Autodesk Inventor part; units mm, degrees
ref_plane "YZ Plane" through (0, 0, 0) normal (1, 0, 0) x (0, 1, 0)
ref_plane "XZ Plane" through (0, 0, 0) normal (0, 1, 0) x (-1, 0, 0)
ref_plane "XY Plane" through (0, 0, 0) normal (0, 0, 1) x (1, 0, 0)
sketch "Náčrt2" plane through (0, 0, 0) normal (0, 0, 1) x (1, 0, 0)
  line L0 (-2.8, -6) -> (2.8, -6)
  line L1 (2.8, -6) -> (2.8, 6)
  line L2 (2.8, 6) -> (-2.8, 6)
  line L3 (-2.8, 6) -> (-2.8, -6)
  line L4 (-2.8, -6) -> (2.8, 6) construction
  line L5 (2.8, -6) -> (-2.8, 6) construction
  circle A0 centre (0, 0) radius 1.5
  dimension "d0" = 5.6
  dimension "d1" = 12
  dimension "d2" = 3
extrude "Vysunutí1" add sketch "Náčrt2" along normal blind 2.75
fillet "Zaoblení1" radius 1.2 4 edges at (-2.8, 6, 1.375) (2.8, 6, 1.375) (2.8, -6, 1.375) (-2.8, -6, 1.375)
chamfer "Zkosení1" distance 0.2 angle 45 2 edges at (-1.5, 0, 2.75) (-1.5, 0, 0)
properties part number "rapoukServoWasherv0_3D tisk"
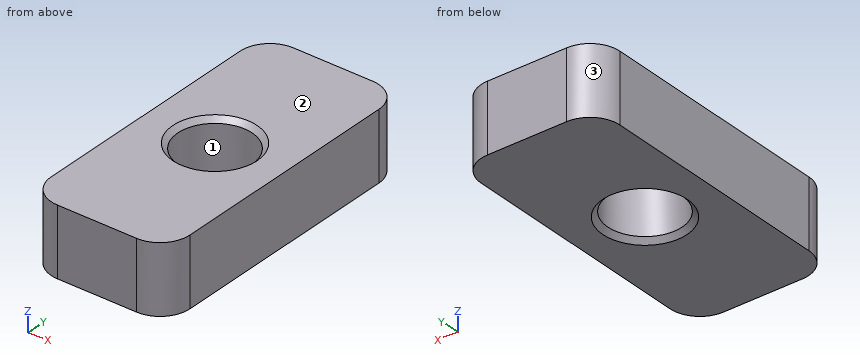
Check sheet for the modelled part. Datum: model origin and axes. Units: mm. Face numbers are marked on the shaded views. Round coordinates to 2 decimals unless told otherwise and drop trailing zeros. Loops run counter-clockwise (first coordinate to the right, second up) from the corner with the lowest first, then second, coordinate; pieces in that order, holes last. Notation, with made-up numbers: M -12,68.25 L 36,68.25 A26 ccw 36,82.25 Z; hole C -28,23 d8. An arc over 180 degrees is marked long. Answer as a JSON object with one key per item and string values.
1. Section check C-C (z = 1). Record the boundary of the cut face in (x, y), plus the area to 3 significant figures.
Reply:
{"outline": "M -2.8,-4.8 A1.2 ccw -1.6,-6 L 1.6,-6 A1.2 ccw 2.8,-4.8 L 2.8,4.8 A1.2 ccw 1.6,6 L -1.6,6 A1.2 ccw -2.8,4.8 Z; hole C 0,0 d3", "area": "58.9 mm²"}
2. Mould release check, pull along Y, two halves, no side actions. Record for the marked faces 1, 2 and 3: pulls with the +Y half, pulls with the -Y half, needs draft (parallel to the pull), parting line crosses it, or undercut.
Reply:
{"face 1": "undercut", "face 2": "needs draft", "face 3": "pulls with the +Y half"}
3. Section check B-B (y = 0). Record the boundary of the cut face in (x, z), plus the area to 3 significant figures.
Reply:
{"outline": "M -2.8,0 L -1.7,0 L -1.5,0.2 L -1.5,2.55 L -1.7,2.75 L -2.8,2.75 Z; M 1.5,0.2 L 1.7,0 L 2.8,0 L 2.8,2.75 L 1.7,2.75 L 1.5,2.55 Z", "area": "7.07 mm²"}
4. Section check A-A (x = 0). Record the boundary of the cut face in (y, z).
Reply:
{"outline": "M -6,0 L -1.7,0 L -1.5,0.2 L -1.5,2.55 L -1.7,2.75 L -6,2.75 Z; M 1.5,0.2 L 1.7,0 L 6,0 L 6,2.75 L 1.7,2.75 L 1.5,2.55 Z"}
5. Scan lines: line 1 (Y direction, x = 0, z = 1.7); line 2 (Y direction, x = 0.9, z = 2.3); line 3 (X direction, y = 1.25, z = 0.3). Record each from-to range of solid material in increasing order.
Reply:
{"line 1": "y = -6 to -1.5, 1.5 to 6", "line 2": "y = -6 to -1.2, 1.2 to 6", "line 3": "x = -2.8 to -0.83, 0.83 to 2.8"}
